from build123d import *

# Parameters (mm, degrees)
F0_W     = 15.546926
F0_H     = 3.734995
F1_DEPTH = 7.62


with BuildPart() as f1:
    # F0 (on Front) → F1 (new body)
    with BuildSketch(Plane.XZ):
        with BuildLine():
            ThreePointArc((76.2, 36.83), (73.968154, 42.218154), (68.58, 44.45))
            Line((68.58, 44.45), (-68.58, 44.45))
            ThreePointArc((-68.58, 44.45), (-73.968154, 42.218154), (-76.2, 36.83))
            Line((-76.2, 36.83), (-76.2, 10.266046))
            Line((-76.2, 10.266046), (-76.2, -36.83))
            ThreePointArc((-76.2, -36.83), (-73.968154, -42.218154), (-68.58, -44.45))
            Line((-68.58, -44.45), (68.58, -44.45))
            ThreePointArc((68.58, -44.45), (73.968154, -42.218154), (76.2, -36.83))
            Line((76.2, -36.83), (76.2, -27.426558))
            Line((76.2, -27.426558), (76.2, -23.691563))
            Line((76.2, -23.691563), (76.2, 8.486843))
            Line((76.2, 8.486843), (56.458235, 8.486843))
            Line((56.458235, 8.486843), (56.458235, -7.602361))
            Line((56.458235, -7.602361), (48.076235, -7.602361))
            Line((48.076235, -7.602361), (48.076235, 8.486843))
            Line((48.076235, 8.486843), (48.076235, 16.868843))
            Line((48.076235, 16.868843), (56.458235, 16.868843))
            Line((56.458235, 16.868843), (76.2, 16.868843))
            Line((76.2, 16.868843), (76.2, 36.83))
        make_face()
        with BuildLine():
            ThreePointArc((-60.96, -36.83), (-63.5, -39.37), (-66.04, -36.83))
            ThreePointArc((-66.04, -36.83), (-63.5, -34.29), (-60.96, -36.83))
        make_face(mode=Mode.SUBTRACT)
        with BuildLine():
            ThreePointArc((-48.26, -36.83), (-50.8, -39.37), (-53.34, -36.83))
            ThreePointArc((-53.34, -36.83), (-50.8, -34.29), (-48.26, -36.83))
        make_face(mode=Mode.SUBTRACT)
        with BuildLine():
            ThreePointArc((-35.56, -36.83), (-38.1, -39.37), (-40.64, -36.83))
            ThreePointArc((-40.64, -36.83), (-38.1, -34.29), (-35.56, -36.83))
        make_face(mode=Mode.SUBTRACT)
        with BuildLine():
            ThreePointArc((-22.86, -36.83), (-25.4, -39.37), (-27.94, -36.83))
            ThreePointArc((-27.94, -36.83), (-25.4, -34.29), (-22.86, -36.83))
        make_face(mode=Mode.SUBTRACT)
        with BuildLine():
            ThreePointArc((-10.16, -36.83), (-12.7, -39.37), (-15.24, -36.83))
            ThreePointArc((-15.24, -36.83), (-12.7, -34.29), (-10.16, -36.83))
        make_face(mode=Mode.SUBTRACT)
        with BuildLine():
            ThreePointArc((2.54, -36.83), (0, -39.37), (-2.54, -36.83))
            ThreePointArc((-2.54, -36.83), (0, -34.29), (2.54, -36.83))
        make_face(mode=Mode.SUBTRACT)
        with BuildLine():
            ThreePointArc((29.386759, -31.245217), (25.576759, -35.055217), (21.766759, -31.245217))
            Line((21.766759, -31.245217), (21.766759, -21.085217))
            ThreePointArc((21.766759, -21.085217), (25.576759, -17.275217), (29.386759, -21.085217))
            Line((29.386759, -21.085217), (29.386759, -31.245217))
        make_face(mode=Mode.SUBTRACT)
        with BuildLine():
            ThreePointArc((-60.325, 10.266046), (-64.77, 5.821046), (-69.215, 10.266046))
            ThreePointArc((-69.215, 10.266046), (-64.77, 14.711046), (-60.325, 10.266046))
        make_face(mode=Mode.SUBTRACT)
        with BuildLine():
            ThreePointArc((-38.735, 10.266046), (-43.18, 5.821046), (-47.625, 10.266046))
            ThreePointArc((-47.625, 10.266046), (-43.18, 14.711046), (-38.735, 10.266046))
        make_face(mode=Mode.SUBTRACT)
        with BuildLine():
            ThreePointArc((-17.145, 10.266046), (-21.59, 5.821046), (-26.035, 10.266046))
            ThreePointArc((-26.035, 10.266046), (-21.59, 14.711046), (-17.145, 10.266046))
        make_face(mode=Mode.SUBTRACT)
        with BuildLine():
            ThreePointArc((4.445, 10.266046), (0, 5.821046), (-4.445, 10.266046))
            ThreePointArc((-4.445, 10.266046), (0, 14.711046), (4.445, 10.266046))
        make_face(mode=Mode.SUBTRACT)
        with Locations((83.973463, -25.559061)):
            Rectangle(F0_W, F0_H)
    extrude(amount=F1_DEPTH)


solid = f1.part
Can you work these out from the model? Positions are in its coordinate system, mm. A direction names the side the tool comes from. Round coordinates to 2 decimals unless told otherwise and drop trailing zeros. Loops run counter-clockwise (first coordinate to the right, second up) from the corner with the lowest first, then second, coordinate; pieces in that order, holes last. Notation, with made-up numbers: (-32, 51) - (8, 51) arc R5 cw to (8, 59) - close; hole circle Ø4 at (-35, 55.5). An arc over 180 degrees is marked (long way). Answer in a Markdown table with one row per item. Add a question column.
Q1. For pin 1 Ø8 at (x, z) = (-50.8, -36.83) entering from -Y; pin 2 Ø1.5 at (y, z) = (-1.5, -35) entering from +X, each with a flat end and sliding along its axis, tell me the tip position at first contact or that it passes through.
Q2. I want a section at B-B on x = 58. List the corners of the cut face in (y, z) for me, and give its area (3 significant figures).
Q3. Which directions (+Z, -Z, +X, -X, +Y, -Y) give clear straight access to the entire face, cutting with the end or side of a thin tool? Please do faces 5 (the flat face through (84, -4, -27.427)), 6 (the cylindrical face through (25.661, -3.757, -35.054)), 7 (the flat face through (91.747, -4, -26)).
Q4. I want a section at C-C on y = -2.5. Count the separate pieces of the cut face and the enclosed holes in it, and give its area (3 significant figures).
Q5. We'd pull the mould along Z, two halves only. Please class faces 1 (the cylindrical face through (-73.909, -3.757, 42.277)), 2 (the flat face through (62, -4, 16.869)), 3 (the flat face through (-12, 0, 1)), 4 (the flat face through (52, -4, -7.602)): pulls with the +Z half, pulls with the -Z half, needs draft (parallel to the pull), parting line crosses it, or undercut.
Q6. I want a section at A-A on x = 0. List the corners of the cut face in (y, z) for me, and give its area (3 significant figures).
Q7. I want a section at D-D on z = 30. List the corners of the cut face in (x, y) for me, and give its area (3 significant figures).
Q8. I need wall thicknesses on L1, parallel to Z at x = -21.59, y = -6; L2, parallel to Z at x = 0, y = -4.5; L3, parallel to Z at x = -64.77, y = -5.75. Which ranges of each line are inside material? Lowest first, please.
A:
| question | item | result |
|---|---|---|
| 1 | pin 1 | y = -7.62 |
| 1 | pin 2 | x = 76.2 |
| 2 | outline | (-7.62, -44.45) - (0, -44.45) - (0, 8.49) - (-7.62, 8.49) - close; (-7.62, 16.87) - (0, 16.87) - (0, 44.45) - (-7.62, 44.45) - close |
| 2 | area | 614 mm^2 |
| 3 | face 5 | -Z, +X, +Y, -Y |
| 3 | face 6 | +Y, -Y |
| 3 | face 7 | +Z, -Z, +X, +Y, -Y |
| 4 | separate pieces | 1 |
| 4 | enclosed holes | 11 |
| 4 | area | 12,700 mm^2 |
| 5 | face 1 | pulls with the +Z half |
| 5 | face 2 | undercut |
| 5 | face 3 | needs draft |
| 5 | face 4 | undercut |
| 6 | outline | (-7.62, -44.45) - (0, -44.45) - (0, -39.37) - (-7.62, -39.37) - close; (-7.62, -34.29) - (0, -34.29) - (0, 5.82) - (-7.62, 5.82) - close; (-7.62, 14.71) - (0, 14.71) - (0, 44.45) - (-7.62, 44.45) - close |
| 6 | area | 571 mm^2 |
| 7 | outline | (-76.2, -7.62) - (76.2, -7.62) - (76.2, 0) - (-76.2, 0) - close |
| 7 | area | 1,160 mm^2 |
| 8 | L1 | -44.45 to 5.82, 14.71 to 44.45 |
| 8 | L2 | -44.45 to -39.37, -34.29 to 5.82, 14.71 to 44.45 |
| 8 | L3 | -44.45 to -39.03, -34.63 to 5.82, 14.71 to 44.45 |
